For this review, take the finished solid that the model builds, in its own axes (mm). A direction names the side the tool comes from. Round coordinates to 2 decimals unless told otherwise and drop trailing zeros. Write each loop counter-clockwise with the first axis right and the second up, starting at its lowest first coordinate (ties: lowest second). Pieces come first, ordered by that corner, then holes. Notation, with made-up numbers: M 14,-27.5 L 47,-27.5 A28 cw 47,-8.5 Z; hole C -1,39.25 d4. An arc over 180 degrees is marked long. Answer in a Markdown table with one row per item.
```python
from build123d import *

# Parameters (mm, degrees)
CROQUIS1_R              = 9.75
CROQUIS1_R_2            = 1.5
CROQUIS1_R_3            = 0.8
SALIENTE_EXTRUIR1_DEPTH = 2
CROQUIS1_3_R            = 3.75
CROQUIS1_3_R_2          = 1.5
SALIENTE_EXTRUIR2_DEPTH = 2.5
CROQUIS2_R              = 4.4
CORTAR_EXTRUIR3_DEPTH   = 3.8
CROQUIS2_6_R            = 4.4
CROQUIS2_6_R_2          = 3.75
SALIENTE_EXTRUIR3_DEPTH = 0.5
CROQUIS2_9_R            = 2.5
CORTAR_EXTRUIR4_DEPTH   = 3.8


with BuildPart() as part:
    # Croquis1 → Saliente-Extruir1 (new body, symmetric)
    with BuildSketch(Plane(origin=(0, 0, 0), x_dir=(1, 0, 0), z_dir=(0, 1, 0))):
        Circle(CROQUIS1_R)
        Circle(CROQUIS1_R_2, mode=Mode.SUBTRACT)
        with Locations((6.75, 0)):
            Circle(CROQUIS1_R_3, mode=Mode.SUBTRACT)
        with Locations((0, -6.75)):
            Circle(CROQUIS1_R_3, mode=Mode.SUBTRACT)
        with Locations((-6.75, 0)):
            Circle(CROQUIS1_R_3, mode=Mode.SUBTRACT)
        with Locations((0, 6.75)):
            Circle(CROQUIS1_R_3, mode=Mode.SUBTRACT)
        with Locations((4.772970773, -4.772970773)):
            Circle(CROQUIS1_R_3, mode=Mode.SUBTRACT)
        with Locations((-4.772970773, -4.772970773)):
            Circle(CROQUIS1_R_3, mode=Mode.SUBTRACT)
        with Locations((-4.772970773, 4.772970773)):
            Circle(CROQUIS1_R_3, mode=Mode.SUBTRACT)
        with Locations((4.772970773, 4.772970773)):
            Circle(CROQUIS1_R_3, mode=Mode.SUBTRACT)
    extrude(amount=SALIENTE_EXTRUIR1_DEPTH, both=True)

    # Croquis1_3 → Saliente-Extruir2 (add, symmetric)
    with BuildSketch(Plane(origin=(0, 0, 0), x_dir=(1, 0, 0), z_dir=(0, 1, 0))):
        Circle(CROQUIS1_3_R)
        Circle(CROQUIS1_3_R_2, mode=Mode.SUBTRACT)
    extrude(amount=SALIENTE_EXTRUIR2_DEPTH, both=True)

    # Croquis2 → Cortar-Extruir3 (cut)
    with BuildSketch(Plane.XZ.offset(2)):
        with BuildLine():
            ThreePointArc((8.493703704, -0.979539378), (4.75, 0), (8.493703704, 0.979539378))
            ThreePointArc((8.493703704, 0.979539378), (7.899170003, 3.271943347), (6.698594423, 5.313316549))
            ThreePointArc((6.698594423, 5.313316549), (6.754289437, 5.045691051), (6.772970773, 4.772970773))
            ThreePointArc((6.772970773, 4.772970773), (3.179124552, 3.564809267), (5.313316549, 6.698594423))
            ThreePointArc((5.313316549, 6.698594423), (3.271943347, 7.899170003), (0.979539378, 8.493703704))
            ThreePointArc((0.979539378, 8.493703704), (1.72613423, 7.76017851), (2, 6.75))
            ThreePointArc((2, 6.75), (-1.01017851, 5.02386577), (-0.979539378, 8.493703704))
            ThreePointArc((-0.979539378, 8.493703704), (-3.271943347, 7.899170003), (-5.313316549, 6.698594423))
            ThreePointArc((-5.313316549, 6.698594423), (-3.564809267, 6.366816994), (-2.772970773, 4.772970773))
            ThreePointArc((-2.772970773, 4.772970773), (-5.045691051, 2.791652109), (-6.698594423, 5.313316549))
            ThreePointArc((-6.698594423, 5.313316549), (-7.899170003, 3.271943347), (-8.493703704, 0.979539378))
            ThreePointArc((-8.493703704, 0.979539378), (-6.243742856, 1.934865293), (-4.75, 0))
            ThreePointArc((-4.75, 0), (-6.243742856, -1.934865293), (-8.493703704, -0.979539378))
            ThreePointArc((-8.493703704, -0.979539378), (-7.899170003, -3.271943347), (-6.698594423, -5.313316549))
            ThreePointArc((-6.698594423, -5.313316549), (-5.045691051, -2.791652109), (-2.772970773, -4.772970773))
            ThreePointArc((-2.772970773, -4.772970773), (-3.564809267, -6.366816994), (-5.313316549, -6.698594423))
            ThreePointArc((-5.313316549, -6.698594423), (-3.271943347, -7.899170003), (-0.979539378, -8.493703704))
            ThreePointArc((-0.979539378, -8.493703704), (-1.01017851, -5.02386577), (2, -6.75))
            ThreePointArc((2, -6.75), (1.72613423, -7.76017851), (0.979539378, -8.493703704))
            ThreePointArc((0.979539378, -8.493703704), (3.271943347, -7.899170003), (5.313316549, -6.698594423))
            ThreePointArc((5.313316549, -6.698594423), (3.179124552, -3.564809267), (6.772970773, -4.772970773))
            ThreePointArc((6.772970773, -4.772970773), (6.754289437, -5.045691051), (6.698594423, -5.313316549))
            ThreePointArc((6.698594423, -5.313316549), (7.899170003, -3.271943347), (8.493703704, -0.979539378))
        make_face()
        Circle(CROQUIS2_R, mode=Mode.SUBTRACT)
    extrude(amount=-CORTAR_EXTRUIR3_DEPTH, mode=Mode.SUBTRACT)

    # Croquis2_6 → Saliente-Extruir3 (add)
    with BuildSketch(Plane.XZ.offset(2)):
        Circle(CROQUIS2_6_R)
        Circle(CROQUIS2_6_R_2, mode=Mode.SUBTRACT)
    extrude(amount=SALIENTE_EXTRUIR3_DEPTH)

    # Croquis2_9 → Cortar-Extruir4 (cut, symmetric)
    with BuildSketch(Plane.XZ.offset(2)):
        Circle(CROQUIS2_9_R)
    extrude(amount=CORTAR_EXTRUIR4_DEPTH, both=True, mode=Mode.SUBTRACT)


solid = part.part
```
Q1. Take a section at A-A (y = 0.1). State how many separate pieces and enclosed holes the cut face has, then the cut area to 3 significant figures.
Found:
| item | result |
|---|---|
| separate pieces | 2 |
| enclosed holes | 10 |
| area | 192 mm² |
Q2. Mouldability with a two-part tool opening along X and no side actions: class faces 4 (the face through (2, 2.5, 0)), 5 (the face through (-7.912, -0.127, -3.241)), 6 (the face through (-1.269, 0.028, -9.667)), 7 (the face through (-0.54, -0.38, -2.44)) as +X half, -X half, draft (parallel to the pull), parting line (faces both ways), or undercut.
Found:
| item | result |
|---|---|
| face 4 | draft |
| face 5 | undercut |
| face 6 | parting line |
| face 7 | undercut |
Q3. Insertion check: P1, Ø6, axis at x = 0, z = 0, coming from the +Y side; P2, Ø2, axis at x = -4.77, z = 4.77, coming from the +Y side; P3, Ø2, axis at x = 5, y = 1, coming from the +Z side; P4, Ø2, axis at x = 0, z = 6.75, coming from the -Y side. Each pin has a flat end and moves straight along its axis. Give the tip position at first contact, or say it passes through.
Found:
| item | result |
|---|---|
| P1 | y = 2.5 |
| P2 | y = 2 |
| P3 | z = 8.89 |
| P4 | y = -2 |
Q4. For probe 1 along Z at (x, y) = (0, 0.3); probe 2 along Z at (x, y) = (3, -0.95), list the stretches that pass through material, from the lowest coordinate up.
Found:
| item | result |
|---|---|
| probe 1 | -9.75 to -7.55, -5.95 to -4.75, -4.4 to -2.5, 2.5 to 4.4, 4.75 to 5.95, 7.55 to 9.75 |
| probe 2 | -9.28 to -8.01, -5.7 to -3.85, -3.22 to 3.22, 3.85 to 5.7, 8.01 to 9.28 |
Q5. Take a section at D-D (z = -1.75). State the section outline as (x, y) points.
Found:
| item | result |
|---|---|
| outline | M -9.59,-2 L -8.37,-2 L -8.37,1.8 L -7.72,1.8 L -7.72,-2 L -5.78,-2 L -5.78,1.8 L -4.04,1.8 L -4.04,-2.5 L -1.79,-2.5 L -1.79,1.8 L 1.79,1.8 L 1.79,-2.5 L 4.04,-2.5 L 4.04,1.8 L 5.78,1.8 L 5.78,-2 L 7.72,-2 L 7.72,1.8 L 8.37,1.8 L 8.37,-2 L 9.59,-2 L 9.59,2 L 3.32,2 L 3.32,2.5 L -3.32,2.5 L -3.32,2 L -9.59,2 Z |
Q6. Machinability: for faces 1 (the face through (0, -2, 5)), 2 (the face through (-1.5, 2.15, -0.07)), 3 (the face through (-3.746, 2.254, -0.165)), which of the approach directions +Z, -Z, +X, -X, +Y, -Y give a long, thin tool a straight path to every point of the face, cutting with its end or side? Answer none if there is none.
Found:
| item | result |
|---|---|
| face 1 | -Y |
| face 2 | +Y, -Y |
| face 3 | +Y |
